The model under review builds one solid part; all positions refer to its coordinate system, in mm. Face numbers are marked on the shaded views. A direction names the side the tool comes from. Coordinates: 2 decimals unless noted, no trailing zeros. Write each loop counter-clockwise with the first axis right and the second up, starting at its lowest first coordinate (ties: lowest second). Pieces come first, ordered by that corner, then holes.
```python
from build123d import *

# Parameters (mm, degrees)
SKETCH_1_R          = 4.15
EXTRUDE_1_DEPTH     = 3
EXTRUDE_2_DEPTH     = 12
CUT_EXTRUDE_1_DEPTH = 112.858735101


with BuildPart() as part:
    # 草图1 → 凸台-拉伸1 (new body)
    with BuildSketch(Plane(origin=(0, 0, 0), x_dir=(1, 0, 0), z_dir=(0, 1, 0))):
        with BuildLine():
            ThreePointArc((19.532394726, 15.60402372), (-17.67766953, 17.67766953), (-15.60402372, -19.532394726))
            Line((-15.60402372, -19.532394726), (54.277196075, -75.359047143))
            ThreePointArc((54.277196075, -75.359047143), (74.246212025, -74.246212025), (75.359047143, -54.277196075))
            Line((75.359047143, -54.277196075), (19.532394726, 15.60402372))
        make_face()
        with Locations(Location((0, 0, 0), (0, 0, 270))):
            Circle(SKETCH_1_R, mode=Mode.SUBTRACT)
        with Locations(Location((63.639610307, -63.639610307, 0), (0, 0, 270))):
            Circle(SKETCH_1_R, mode=Mode.SUBTRACT)
    extrude(amount=EXTRUDE_1_DEPTH)

    # 草图3 → 凸台-拉伸2 (add)
    with BuildSketch(Plane(origin=(0, 3, 0), x_dir=(1, 0, 0), z_dir=(0, 1, 0))):
        with BuildLine():
            ThreePointArc((54.277196075, -75.359047143), (74.246212025, -74.246212025), (75.359047143, -54.277196075))
            Line((75.359047143, -54.277196075), (19.532394726, 15.60402372))
            ThreePointArc((19.532394726, 15.60402372), (-17.67766953, 17.67766953), (-15.60402372, -19.532394726))
            Line((-15.60402372, -19.532394726), (54.277196075, -75.359047143))
        make_face()
        with BuildLine():
            Line((17.969803148, 14.355701822), (73.796455565, -55.525517972))
            ThreePointArc((73.796455565, -55.525517972), (72.831998462, -72.831998462), (55.525517972, -73.796455565))
            Line((55.525517972, -73.796455565), (-14.355701822, -17.969803148))
            ThreePointArc((-14.355701822, -17.969803148), (-16.263455967, 16.263455967), (17.969803148, 14.355701822))
        make_face(mode=Mode.SUBTRACT)
    extrude(amount=EXTRUDE_2_DEPTH)

    # 草图4 → 切除-拉伸1 (cut, through all)
    with BuildSketch(Plane(origin=(0, 3, 0), x_dir=(1, 0, 0), z_dir=(0, 1, 0))):
        Polygon((17.133662373, -2.976992155), (10.055327264, -10.055327264), (54.909619217, -54.909619217), (61.987954325, -47.831284108), align=None)
        Polygon((54.909619217, -54.909619217), (10.055327264, -10.055327264), (2.529939412, -17.580715117), (47.384231364, -62.435007069), align=None)
    extrude(amount=-CUT_EXTRUDE_1_DEPTH, mode=Mode.SUBTRACT)


solid = part.part
```
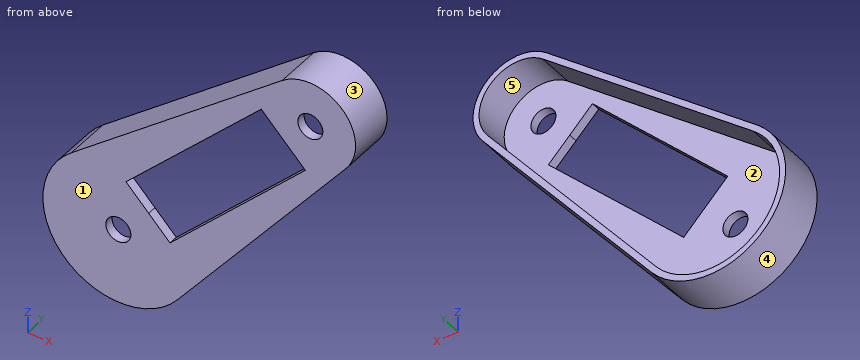
Item 1: Take a section at B-B, the plane z = 58. Write out the cut boundary in (x, y).
Solved:
outline: (32.55, 0) - (42.95, 0) - (42.95, 3) - (35.75, 3) - (35.75, 15) - (32.55, 15) - close; (51.82, 0) - (77.54, 0) - (77.54, 15) - (75.35, 15) - (75.35, 3) - (51.82, 3) - close
Item 2: To check wall thickness, follow line 1 along Y through (x, z) = (19, 41.5); line 2 along Z through (x, y) = (46, 11.5); line 3 along Z through (x, y) = (-14.5, 8.75). State the ranges of each line that lie inside material, in increasing order.
Solved:
line 1: y = 0 to 3
line 2: z = 17.53 to 20.73, 66.19 to 68.75
line 3: z = -20.37 to -17.85, 17.85 to 20.41
Item 3: For pin 1 (8 mm diameter, centred on x = 33.5, y = 12.5, fed in from +Z); pin 2 (1.5 mm diameter, centred on x = 29, z = 46.5, fed in from +Y); pin 3 (1.5 mm diameter, centred on x = 38.5, y = 2.5, fed in from +Z); pin 4 (7.5 mm diameter, centred on x = 63.64, z = 63.64, fed in from +Y), all flat-tipped, find the tip position at first contact; note any pin that passes through.
Solved:
pin 1: stops at z = 61.96
pin 2: stops at y = 3
pin 3: stops at z = 63.35
pin 4: passes through
Item 4: Take a section at D-D, the plane z = -11. Write out the cut boundary in (x, y).
Solved:
outline: (-22.45, 0) - (23.21, 0) - (23.21, 15) - (20.65, 15) - (20.65, 3) - (-20.2, 3) - (-20.2, 15) - (-22.45, 15) - close
Item 5: Take a section at C-C, the plane x = 0. Write out the cut boundary in (y, z), plus the area to 3 significant figures.
Solved:
outline: (0, -25) - (15, -25) - (15, -23) - (3, -23) - (3, -4.15) - (0, -4.15) - close; (0, 4.15) - (3, 4.15) - (3, 29.44) - (15, 29.44) - (15, 32) - (0, 32) - close
area: 201 mm2
Item 6: Mouldability with a two-part tool opening along Z and no side actions: class the marked faces 1, 2 and 3 as pulls with the +Z half, pulls with the -Z half, needs draft (parallel to the pull), parting line crosses it, or undercut.
Solved:
face 1: needs draft
face 2: undercut
face 3: parting line crosses it
Item 7: Machinability: for the marked faces 4 and 5, which of the approach directions +Z, -Z, +X, -X, +Y, -Y give a long, thin tool a straight path to every point of the face, cutting with its end or side? Answer none if there is none.
Solved:
face 4: +Y, -Y
face 5: +Y
Item 8: Take a section at A-A, the plane y = 13.75. Write out the cut boundary in (x, z).
Solved:
outline: (-15.6, 19.53) arc R25 ccw (long way) to (19.53, -15.6) - (75.36, 54.28) arc R15 ccw to (54.28, 75.36) - close; hole (-14.36, 17.97) arc R23 ccw (long way) to (17.97, -14.36) - (73.8, 55.53) arc R13 ccw to (55.53, 73.8) - close
